```python
from build123d import *

# Parameters (mm, degrees)
EXTRUDE_THIN6_DEPTH = 257
CUT_EXTRUDE1_DEPTH  = 261.716320931


with BuildPart() as part:
    # Sketch2 → Extrude-Thin6 (new body)
    with BuildSketch(Plane.XY):
        Polygon((30, 0), (0, 0), (0, 30), (-2, 30), (-2, -2), (30, -2), align=None)
    extrude(amount=EXTRUDE_THIN6_DEPTH)

    # Sketch3 → Cut-Extrude1 (cut, through all)
    with BuildSketch(Plane(origin=(0, -2, 0), x_dir=(1, 0, 0), z_dir=(0, 1, 0))):
        Polygon((-2, 0), (30, -32), (30, 0), align=None)
        Polygon((30, -257), (30, -225), (-2, -257), align=None)
    extrude(amount=CUT_EXTRUDE1_DEPTH, mode=Mode.SUBTRACT)


solid = part.part
```
The listing builds one solid part. Answer for the finished solid, in the listing's coordinates (mm). A direction names the side the tool comes from. Give positions to 0.01 mm unless a question says otherwise; leave off trailing zeros. Loops run counter-clockwise (first coordinate to the right, second up) from the corner with the lowest first, then second, coordinate; pieces in that order, holes last. Notation, with made-up numbers: M 29.5,51.25 L 56.5,51.25 A18 ccw 56.5,57.25 Z; hole C 5.5,-13 d3. An arc over 180 degrees is marked long. One line per item, written item: value.
Q1. A cutting plane is placed at B-B on x = 9.5. Determine the outline of the cut face in (y, z).
Working result:
outline: M -2,11.5 L 0,11.5 L 0,245.5 L -2,245.5 Z
Q2. A cutting plane is placed at A-A on z = 79. Determine the outline of the cut face in (x, y), then the cut area to 3 significant figures.
Working result:
outline: M -2,-2 L 30,-2 L 30,0 L 0,0 L 0,30 L -2,30 Z
area: 124 mm^2
Q3. A cutting plane is placed at C-C on y = 17.5. Determine the outline of the cut face in (x, z).
Working result:
outline: M -2,0 L 0,2 L 0,255 L -2,257 Z
Q4. Find the intervals of material crossed by line 1 (Y direction, x = 0.5, z = 245.5), in increasing order. Write a range as from..to.
Working result:
line 1: y = -2..0
Q5. For faces 1 (the face through (0, 15, 127)), 2 (the face through (6.8, -0.3, 8.8)), determine the directions among +Z, -Z, +X, -X, +Y, -Y from which every point of the face is accessible in a straight line to the end or side of a thin tool.
Working result:
face 1: +Z, -Z, +X, +Y
face 2: -Z, +X, +Y, -Y
Q6. A cutting plane is placed at D-D on z = 27. Determine the outline of the cut face in (x, y), then the cut area to 3 significant figures.
Working result:
outline: M -2,-2 L 25,-2 L 25,0 L 0,0 L 0,30 L -2,30 Z
area: 114 mm^2
Q7. Flat-ended cylindrical pins translate along their axes: P1, Ø4, axis at y = 17, z = 50, coming from the +X side; P2, Ø6, axis at x = 17, z = 84.5, coming from the +Y side. Find the tip coordinate at first contact, or state that the pin passes through.
Working result:
P1: stops at x = 0
P2: stops at y = 0
